Autodesk Inventor part; units mm, degrees
ref_plane "工作平面1" through (0, 10, 0) normal (0, 1, 0) x (-1, 0, 0)
ref_plane "工作平面2" through (0, -15, 201) normal (0, 1, 0) x (-1, 0, 0)
ref_plane "YZ Plane" through (0, 0, 0) normal (1, 0, 0) x (0, 1, 0)
sketch "草图1" plane through (0, 0, 0) normal (0, 0, 1) x (1, 0, 0)
  circle A0 centre (0, 0) radius 10
  dimension "d0" = 20
extrude "拉伸1" add sketch "草图1" along normal blind 51
sketch "草图2" plane through (0, 0, 51) normal (0, 0, 1) x (1, 0, 0)
  circle A0 centre (0, 0) radius 15
  dimension "d3" = 30
extrude "拉伸2" add sketch "草图2" along normal blind 90
sketch "草图3" plane through (0, 0, 141) normal (0, 0, 1) x (1, 0, 0)
  circle A0 centre (0, 0) radius 20
  dimension "d6" = 40
extrude "拉伸3" add sketch "草图3" along normal blind 60
sketch "草图4" plane through (0, 0, 201) normal (0, 0, 1) x (1, 0, 0)
  circle A0 centre (0, 0) radius 15
  dimension "d9" = 30
extrude "拉伸4" add sketch "草图4" along normal blind 46
chamfer "倒角1" distance 1 angle 45 2 edges at (-15, 0, 247) (-10, 0, 0)
ref_plane "工作平面1" through (0, 10, 0) normal (0, 1, 0) x (-1, 0, 0)
sketch "草图5" plane through (0, 10, 0) normal (0, 1, 0) x (-1, 0, 0)
  line L0 (3, 44.5) -> (-3, 44.5)
  line L1 (-3, 44.5) -> (-3, 22.5)
  line L2 (-3, 22.5) -> (3, 22.5)
  line L3 (3, 22.5) -> (3, 44.5)
  arc A0 (-3, 22.5) -> (3, 22.5) centre (0, 22.5) ccw
  arc A1 (3, 44.5) -> (-3, 44.5) centre (0, 44.5) ccw
  line L4 (0, 0) -> (0, -6.1876)
  line L5 (-15, 51) -> (15, 51)
  dimension "d15" = 6
  dimension "d16" = 6.1876
  dimension "d17" = 6.5
  dimension "d18" = 22
extrude "拉伸5" cut sketch "草图5" against normal blind 2.5
ref_plane "工作平面2" through (0, -15, 201) normal (0, 1, 0) x (-1, 0, 0)
sketch "草图6" plane through (0, -15, 201) normal (0, 1, 0) x (-1, 0, 0)
  line L0 (-4, 23.5) -> (4, 23.5)
  line L1 (4, 23.5) -> (4, 6.5)
  line L2 (4, 6.5) -> (-4, 6.5)
  line L3 (-4, 6.5) -> (-4, 23.5)
  arc A0 (-4, 6.5) -> (4, 6.5) centre (0, 6.5) ccw
  arc A1 (4, 23.5) -> (-4, 23.5) centre (0, 23.5) ccw
  line L4 (20, 0) -> (-20, 0)
  line L5 (0, 0) -> (0, 6.5)
  point P0 (0, -201)
  dimension "d21" = 6.5
  dimension "d22" = 8
  dimension "d23" = 17
extrude "拉伸6" cut sketch "草图6" along normal blind 3
properties part number "齿轮160配件"
The model under review builds one solid part; all positions refer to its coordinate system, in mm. A direction names the side the tool comes from. Round coordinates to 2 decimals unless told otherwise and drop trailing zeros. Loops run counter-clockwise (first coordinate to the right, second up) from the corner with the lowest first, then second, coordinate; pieces in that order, holes last. Notation, with made-up numbers: (-10, 65) - (44, 65) arc R25 ccw to (44, 103) - close; hole circle Ø8 at (4.5, 87). An arc over 180 degrees is marked (long way). Use a Markdown table: item, result. Add a question column.
Q1. Insertion check: pin 1 Ø1.2 at (y, z) = (-13.5, 218) entering from +X; pin 2 Ø2.5 at (x, z) = (1.5, 214) entering from -Y; pin 3 Ø2 at (y, z) = (8.5, 30) entering from +X. Each pin has a flat end and moves straight along its axis. Give the tip position at first contact, or say it passes through.
Q2. For probe 1 along Z at (x, y) = (12, 11); probe 2 along Z at (x, y) = (-4, -11.5); probe 3 along X at (y, z) = (-12.5, 200), list the stretches that pass through material, from the lowest coordinate up.
Q3. Machinability: for faces 1 (the face through (-0.1, -13.5, 203.5)), 2 (the face through (-3.252, 14.643, 223.185)), 3 (the face through (0, 7.5, 34)), which of the approach directions +Z, -Z, +X, -X, +Y, -Y give a long, thin tool a straight path to every point of the face, cutting with its end or side? Answer none if there is none.
Q4. Add section B-B (z = 112). State the section outline as (x, y) points.
Q5. Add section C-C (z = 166.5). State the section outline as (x, y) points, plus the area to 3 significant figures.
Q6. Add section A-A (y = 0). State the section outline as (x, z) points, plus the area to 3 significant figures.
Q7. The part is to be moulded in two halves that separate along Z. For faces 4 (the face through (0, 0, 247)), 5 (the face through (0, -12, 216)), 6 (the face through (3, 15, 141)), say which applies: pulls with the +Z half, pulls with the -Z half, needs draft (parallel to the pull), parting line crosses it, or undercut.
Worked answers:
| question | item | result |
|---|---|---|
| 1 | pin 1 | x = 7.65 |
| 1 | pin 2 | y = -12 |
| 1 | pin 3 | x = 6.61 |
| 2 | probe 1 | 141 to 201 |
| 2 | probe 2 | 51 to 247 |
| 2 | probe 3 | -15.61 to 15.61 |
| 3 | face 1 | -Y |
| 3 | face 2 | +Z |
| 3 | face 3 | +Y |
| 4 | outline | circle Ø30 at (0, 0) |
| 5 | outline | circle Ø40 at (0, 0) |
| 5 | area | 1,260 mm² |
| 6 | outline | (-20, 141) - (-15, 141) - (-15, 51) - (-10, 51) - (-10, 1) - (-9, 0) - (9, 0) - (10, 1) - (10, 51) - (15, 51) - (15, 141) - (20, 141) - (20, 201) - (15, 201) - (15, 246) - (14, 247) - (-14, 247) - (-15, 246) - (-15, 201) - (-20, 201) - close |
| 6 | area | 7,500 mm² |
| 7 | face 4 | pulls with the +Z half |
| 7 | face 5 | undercut |
| 7 | face 6 | pulls with the -Z half |
